Work out the finished part from the listing and answer in its coordinate system (mm). A direction names the side the tool comes from. Round coordinates to 2 decimals unless told otherwise and drop trailing zeros. Loops run counter-clockwise (first coordinate to the right, second up) from the corner with the lowest first, then second, coordinate; pieces in that order, holes last. Notation, with made-up numbers: (-0.75, 87) - (25.25, 87) arc R24 cw to (25.25, 108) - close; hole circle Ø2 at (82, 28). An arc over 180 degrees is marked (long way). Return JSON: item names as keys, results as strings.
from build123d import *

# Parameters (mm, degrees)
F1_DEPTH = 10


with BuildPart() as f1:
    # F0 (on Top) → F1 (new body)
    with BuildSketch(Plane.XY):
        with BuildLine():
            Line((-12.07, 54.529991), (-12.07, 64.529991))
            ThreePointArc((-12.07, 64.529991), (-26.845727, 64.63975), (-37.664252, 54.575273))
            ThreePointArc((-37.664252, 54.575273), (-50.479085, 48.496), (-56.040163, 35.447939))
            ThreePointArc((-56.040163, 35.447939), (-65.447231, 24.83264), (-65.449648, 10.648935))
            ThreePointArc((-65.449648, 10.648935), (-69.94382, -2.803942), (-64.38719, -15.853898))
            ThreePointArc((-64.38719, -15.853898), (-63.249398, -29.991894), (-53.022781, -39.820108))
            ThreePointArc((-53.022781, -39.820108), (-46.435072, -52.381143), (-33.174727, -57.415101))
            ThreePointArc((-33.174727, -57.415101), (-27.219481, -63.87559), (-19.07, -67.160226))
            Line((-19.07, -67.160226), (-19.07, -130.470009))
            add(Edge.make_bspline(
                [(-19.07, -130.470009), (-19.012991, -140.66343), (-41.987017, -140.141293), (-42.07, -145.470009)],
                knots=[0, 0, 0, 0, 27.45906, 27.45906, 27.45906, 27.45906], degree=3))
            Line((-42.07, -145.470009), (-12.07, -145.470009))
            Line((-12.07, -145.470009), (-12.07, -48.521285))
            ThreePointArc((-12.07, -48.521285), (-39.392258, -30.793668), (-50, 0))
            ThreePointArc((-50, 0), (-39.585008, 33.212215), (-12.07, 54.529991))
        make_face()
    extrude(amount=F1_DEPTH)


solid = f1.part
1) A tool of negligible diameter and unlimited length cuts with its end or side. For faces 5 (the cylindrical face through (-39.105, -31.158, 4.93)), 6 (the flat face through (-12.07, -98, 5)), 7 (the cylindrical face through (-27.321, -63.805, 4.93)), from which of +Z, -Z, +X, -X, +Y, -Y can it reach the whole face along a straight path? Write none if from no direction.
Verdict:
{"face 5": "+Z, -Z, +X", "face 6": "+Z, -Z, +X, +Y, -Y", "face 7": "+Z, -Z, -X"}
2) Section A-A (y = -125) is taken. Give the vertices of the cut face in (x, z).
Verdict:
{"outline": "(-19.07, 0) - (-12.07, 0) - (-12.07, 10) - (-19.07, 10) - close"}
3) Find the intervals of material crossed by L1, parallel to Y at x = -20.5, z = 4.25; L2, parallel to Y at x = -29, z = 5; L3, parallel to X at y = -113, z = 0.5, in increasing order.
Verdict:
{"L1": "y = -145.47 to -134.46, -66.87 to -45.6, 50.61 to 65.98", "L2": "y = -145.47 to -139.3, -62.49 to -40.73, 44.74 to 63.65", "L3": "x = -19.07 to -12.07"}
4) Determine the mould class of faces 1 (the cylindrical face through (-50.34, 48.64, 4.93)), 2 (the cylindrical face through (-39.87, 32.8, 4.93)), 3 (the flat face through (-50, -16, 10)), 4 (the flat face through (-27, -145.47, 5)) for opening direction Y: pulls with the +Y half, pulls with the -Y half, needs draft (parallel to the pull), parting line crosses it, or undercut.
Verdict:
{"face 1": "pulls with the +Y half", "face 2": "undercut", "face 3": "needs draft", "face 4": "pulls with the -Y half"}
5) Section C-C (y = -19.5) is taken. Give the vertices of the cut face in (x, z), and give its area (3 significant figures).
Verdict:
{"outline": "(-65.09, 0) - (-46.04, 0) - (-46.04, 10) - (-65.09, 10) - close", "area": "190 mm2"}
6) Flat-ended cylindrical pins translate along their axes: pin 1 (6 mm diameter, centred on y = -116, z = 5, fed in from -X); pin 2 (1 mm diameter, centred on x = -36, z = 1, fed in from +Y); pin 3 (5 mm diameter, centred on x = -49, y = -16.5, fed in from -Z); pin 4 (4 mm diameter, centred on x = -25, y = -40, fed in from +Z). Find the tip coordinate at first contact, or state that the pin passes through.
Verdict:
{"pin 1": "stops at x = -19.07", "pin 2": "stops at y = 58.13", "pin 3": "stops at z = 0", "pin 4": "passes through"}
7) Section B-B (x = -27) is taken. Count the separate pieces of the cut face and the enclosed holes in it, and give its area (3 significant figures).
Verdict:
{"separate pieces": "3", "enclosed holes": "0", "area": "471 mm2"}
